```python
from build123d import *

# Parameters (mm, degrees)
F0_W     = 0.001
F0_H     = 60
F1_DEPTH = 2


# Not quite as in the source:
# - a feature names something its author has since deleted; it is built from what else it names


with BuildPart() as f1:
    # F0 (on Top) → F1 (new body)
    with BuildSketch(Plane.XY):
        Polygon((-409.5329046249, 667.7558401073), (-409.5329046249, 703.2591700554), (-409.5329046249, 710.1822469785), (-439.5329046249, 680.1822469785), (-439.5329046249, 637.7558401073), align=None)
        Polygon((-409.5329046249, 489.3550023332), (-409.5329046249, 667.7558401073), (-439.5329046249, 637.7558401073), (-439.5329046249, 219.3550023332), (-439.5329046249, 189.3550023332), (-439.5329046249, -93.071404538), (-409.5329046249, -63.071404538), (-409.5329046249, -20.6449976668), (-409.5329046249, 189.3550023332), (-409.5329046249, 279.3550023332), (-409.5329046249, 399.3550023332), (-409.5329046249, 459.3550023332), align=None)
        Polygon((-187.1064977537, 489.3550023332), (-409.5329046249, 489.3550023332), (-409.5329046249, 459.3550023332), (-199.5329046249, 459.3550023332), (-157.1064977537, 459.3550023332), align=None)
        Polygon((-499.5329046249, 577.7558401073), (-439.5329046249, 637.7558401073), (-439.5329046249, 680.1822469785), (-499.5329046249, 620.1822469785), (-499.5329046249, 579.3550023332), align=None)
        Polygon((-439.5329046249, 189.3550023332), (-439.5329046249, 219.3550023332), (-857.933742399, 219.3550023332), (-887.933742399, 189.3550023332), align=None)
        Polygon((-529.5329046249, 547.7558401073), (-499.5329046249, 577.7558401073), (-499.5329046249, 579.3550023332), (-499.5329046249, 620.1822469785), (-529.5329046249, 590.1822469785), align=None)
        Polygon((-499.5329046249, 459.3550023332), (-499.5329046249, 577.7558401073), (-529.5329046249, 547.7558401073), (-529.5329046249, 489.3550023332), (-587.933742399, 489.3550023332), (-617.933742399, 459.3550023332), align=None)
        Polygon((-157.1064977537, 459.3550023332), (-199.5329046249, 459.3550023332), (-139.5329046249, 399.3550023332), (40.4670953751, 219.3550023332), (-44.3857183673, 219.3550023332), (-349.5319046249, 219.3550023332), (-349.5329046249, 219.3550023332), (-349.5329046249, 189.3550023332), (-319.5329046249, 189.3550023332), (112.8935022463, 189.3550023332), align=None)
        Polygon((-887.933742399, 189.3550023332), (-857.933742399, 219.3550023332), (-900.3601492702, 219.3550023332), (-930.3601492702, 189.3550023332), align=None)
        Polygon((-900.3601492702, 219.3550023332), (-857.933742399, 219.3550023332), (-797.933742399, 279.3550023332), (-840.3601492702, 279.3550023332), align=None)
        Polygon((-224.3857183673, 399.3550023332), (-349.5329046249, 399.3550023332), (-349.5329046249, 279.3550023332), (-349.5319046249, 279.3550023332), (-104.3857183673, 279.3550023332), align=None)
        Polygon((-677.933742399, 399.3550023332), (-797.933742399, 279.3550023332), (-499.5329046249, 279.3550023332), (-499.5329046249, 399.3550023332), align=None)
        Polygon((-840.3601492702, 279.3550023332), (-797.933742399, 279.3550023332), (-677.933742399, 399.3550023332), (-720.3601492702, 399.3550023332), align=None)
        Polygon((-677.933742399, 399.3550023332), (-617.933742399, 459.3550023332), (-660.3601492702, 459.3550023332), (-720.3601492702, 399.3550023332), align=None)
        Polygon((-660.3601492702, 459.3550023332), (-617.933742399, 459.3550023332), (-587.933742399, 489.3550023332), (-630.3601492702, 489.3550023332), align=None)
        with Locations((-349.5324046249, 249.3550023332)):
            Rectangle(F0_W, F0_H)
        Polygon((-319.5329046249, 26.928595462), (-319.5329046249, 189.3550023332), (-349.5329046249, 189.3550023332), (-349.5329046249, 39.3550023332), (-349.5329046249, -3.071404538), align=None)
        Polygon((-409.5329046249, -20.6449976668), (-409.5329046249, -63.071404538), (-349.5329046249, -3.071404538), (-349.5329046249, 39.3550023332), align=None)
    extrude(amount=F1_DEPTH)


solid = f1.part
```
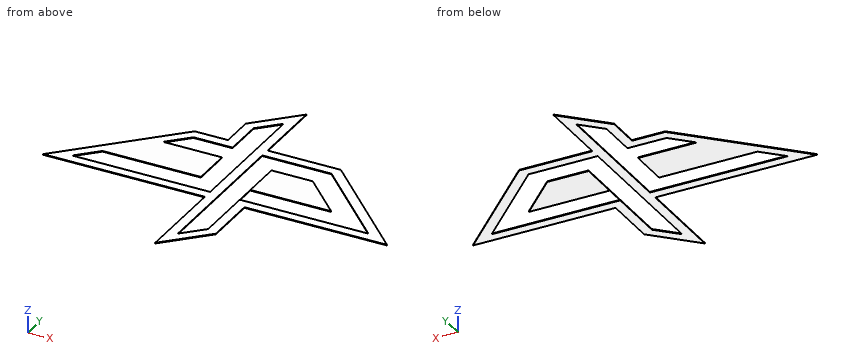
Here's how the part is built. I have some questions about the finished solid (model axes, mm). Coordinates: 2 decimals unless noted, no trailing zeros. Write each loop counter-clockwise with the first axis right and the second up, starting at its lowest first coordinate (ties: lowest second). Pieces come first, ordered by that corner, then holes. Notation, with made-up numbers: M 9.25,11 L 31.25,11 A19 ccw 31.25,43 Z; hole C 82.5,7 d9. An arc over 180 degrees is marked long. Answer as CSV lines item,"result". Start each with the question number.
Q1. Suppose I cut it at B-B, the plane y = 1.5. List the corners of the cut face in (x, z) for me, then the cut area to 3 significant figures.
Q2. Suppose I cut it at C-C, the plane x = -754.5. List the corners of the cut face in (y, z) for me (3 decimals).
Q3. Suppose I cut it at D-D, the plane z = 1.7. State how many separate pieces and enclosed holes the cut face has, then the cut area to 3 significant figures.
Q4. Will these pins go through, and if not, where does the flat tip stop? pin 1 Ø0.6 at (x, z) = (-751, 0.5) entering from +Y; pin 2 Ø1 at (x, z) = (-296.5, 1) entering from -Y (3 decimals); pin 3 Ø1 at (x, z) = (-265.5, 0.5) entering from +Y (3 decimals).
Q5. I need wall thicknesses on probe 1 along Y at (x, z) = (-598, 0.35) (3 decimals); probe 2 along X at (y, z) = (518, 0.4); probe 3 along X at (y, z) = (444.5, 1.95). Which ranges of each line are inside material? Lowest first, please. Write a range as [from, to].
Q6. Suppose I cut it at A-A, the plane x = -283. List the corners of the cut face in (y, z) for me (3 decimals), then the cut area to 3 significant figures.
Entries:
1,outline,"M -439.53,0 L -409.53,0 L -409.53,2 L -439.53,2 Z; M -387.39,0 L -344.96,0 L -344.96,2 L -387.39,2 Z"
1,area,"145 mm²"
2,outline,"M 189.355,0 L 219.355,0 L 219.355,2 L 189.355,2 Z; M 279.355,0 L 365.215,0 L 365.215,2 L 279.355,2 Z"
3,separate pieces,"1"
3,enclosed holes,"2"
3,area,"147,000 mm²"
4,pin 1,"stops at y = 369.02"
4,pin 2,"stops at y = 189.355"
4,pin 3,"stops at y = 489.355"
5,probe 1,"y = [189.355, 219.355], [279.355, 399.355], [459.355, 489.355]"
5,probe 2,"x = [-529.53, -499.53], [-439.53, -409.53]"
5,probe 3,"x = [-675.22, -632.79], [-439.53, -409.53], [-184.68, -142.25]"
6,outline,"M 189.355,0 L 219.355,0 L 219.355,2 L 189.355,2 Z; M 279.355,0 L 399.355,0 L 399.355,2 L 279.355,2 Z; M 459.355,0 L 489.355,0 L 489.355,2 L 459.355,2 Z"
6,area,"360 mm²"
